Check sheet for the drawn part. Datum: minimum x, y, z corner. Units: mm. Round coordinates to 2 decimals unless told otherwise and drop trailing zeros. Write each loop counter-clockwise with the first axis right and the second up, starting at its lowest first coordinate (ties: lowest second). Pieces come first, ordered by that corner, then holes. Notation, with made-up numbers: (29.25, 35) - (84.25, 35) arc R27 ccw to (84.25, 70) - close; hole circle Ø3 at (68, -32). An arc over 180 degrees is marked (long way). Answer as a JSON object with one key per item and string values. Group by question number.
Item 1: Gauge pin test, flat ends, axial feed: P1, Ø8, axis at x = 51.5, z = 21, coming from the +Y side; P2, Ø2, axis at x = 75, z = 14.5, coming from the -Y side; P3, Ø21, axis at x = 58, y = 46, coming from the +Z side; P4, Ø4, axis at x = 54.5, y = 76, coming from the +Z side (3 decimals). Record the tip position at first contact, or that the pin passes through.
Item 2: Sectioned sample at C-C on z = 25. Record the boundary of the cut face in (x, y).
Item 3: Thickness scan on line 1 (X direction, y = 43, z = 13); line 2 (Z direction, x = 19.5, y = 60). Record the ranges inside material, lowest first.
Item 4: Sectioned sample at A-A on x = 43. Record the boundary of the cut face in (y, z) (3 decimals), plus the area to 3 significant figures.
Item 5: Release check for a two-part mould opening along Y. For the marked faces 1, 2, 3 and 4 record: pulls with the +Y half, pulls with the -Y half, needs draft (parallel to the pull), parting line crosses it, or undercut.
Item 6: Sectioned sample at D-D on y = 6. Record the boundary of the cut face in (x, z) (3 decimals), plus the area to 3 significant figures.
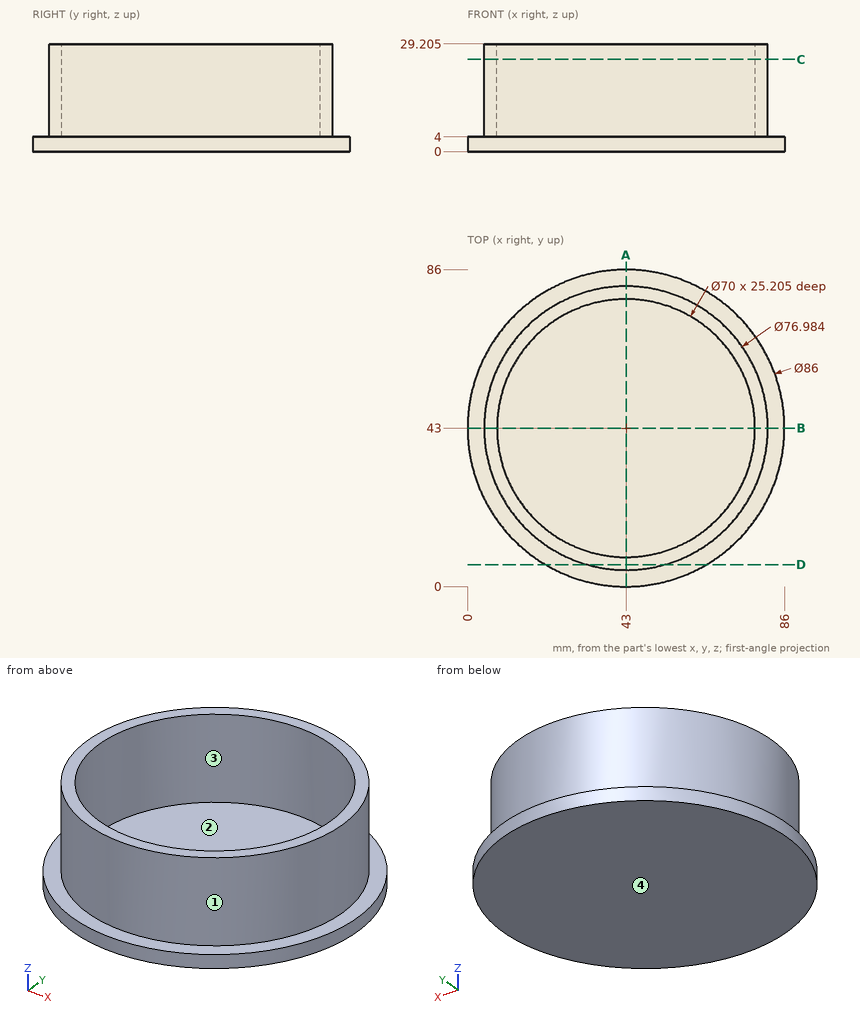
Completed:
{
 "1": {"P1": "y = 81.23", "P2": "y = 20.18", "P3": "z = 4", "P4": "z = 29.205"},
 "2": {"outline": "circle Ø76.98 at (43, 43); hole circle Ø70 at (43, 43)"},
 "3": {"line 1": "4.51 to 8, 78 to 81.49", "line 2": "0 to 4"},
 "4": {"outline": "(0, 0) - (86, 0) - (86, 4) - (81.492, 4) - (81.492, 29.205) - (78, 29.205) - (78, 4) - (8, 4) - (8, 29.205) - (4.508, 29.205) - (4.508, 4) - (0, 4) - close", "area": "520 mm²"},
 "5": {"face 1": "parting line crosses it", "face 2": "undercut", "face 3": "undercut", "face 4": "needs draft"},
 "6": {"outline": "(21.091, 0) - (64.909, 0) - (64.909, 4) - (53.613, 4) - (53.613, 29.205) - (32.387, 29.205) - (32.387, 4) - (21.091, 4) - close", "area": "710 mm²"}
}
